The figure shows three views and two pictorial views of one solid part (mm, origin at its lowest corner). Answer the questions. A direction names the side the tool comes from. Give positions to 0.01 mm unless a question says otherwise; leave off trailing zeros. Loops run counter-clockwise (first coordinate to the right, second up) from the corner with the lowest first, then second, coordinate; pieces in that order, holes last. Notation, with made-up numbers: (73.25, 29) - (103.25, 29) arc R18 cw to (103.25, 51) - close; hole circle Ø10 at (74, 47.25). An arc over 180 degrees is marked (long way). Write each question's results on one line, items separated by ' | '.
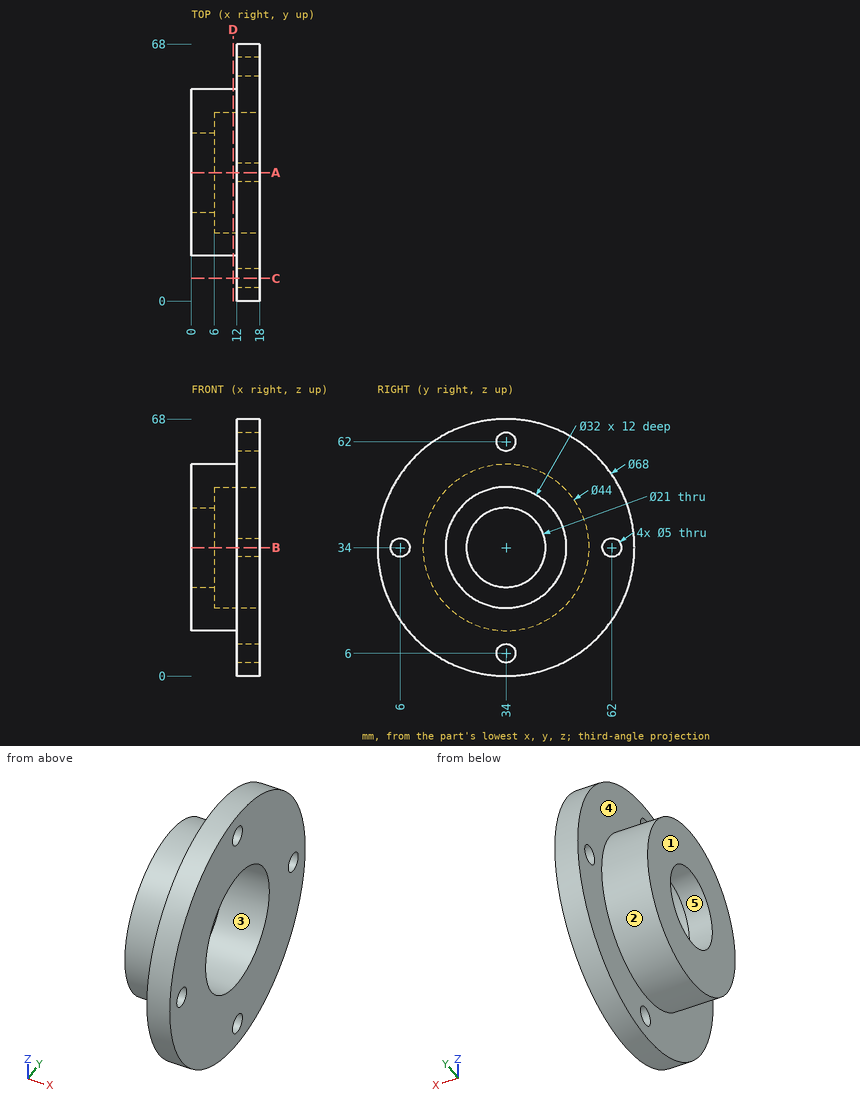
Item 1: Flat-ended cylindrical pins translate along their axes: P1, Ø6, axis at x = 3.5, z = 57, coming from the -Y side; P2, Ø8, axis at x = 6.5, y = 36, coming from the -Z side; P3, Ø1.5, axis at x = 12, y = 44.5, coming from the -Z side; P4, Ø4, axis at y = 6, z = 34, coming from the -X side. Find the tip coordinate at first contact, or state that the pin passes through.
Values found:
P1: stops at y = 24.83 | P2: stops at z = 12 | P3: stops at z = 1.43 | P4: passes through
Item 2: Find the intervals of material crossed by line 1 along Z through (x, y) = (2.25, 34); line 2 along X through (y, z) = (8, 51); line 3 along Y through (x, z) = (12.5, 32.5), in increasing order. Write a range as [from, to].
Values found:
line 1: z = [12, 23.5], [44.5, 56] | line 2: x = [12, 18] | line 3: y = [0.03, 4], [8, 18.07], [49.93, 60], [64, 67.97]
Item 3: A cutting plane is placed at A-A, the plane y = 34. Determine the outline of the cut face in (x, z).
Values found:
outline: (0, 12) - (12, 12) - (12, 8.5) - (18, 8.5) - (18, 18) - (6, 18) - (6, 23.5) - (0, 23.5) - close; (0, 44.5) - (6, 44.5) - (6, 50) - (18, 50) - (18, 59.5) - (12, 59.5) - (12, 56) - (0, 56) - close; (12, 0) - (18, 0) - (18, 3.5) - (12, 3.5) - close; (12, 64.5) - (18, 64.5) - (18, 68) - (12, 68) - close
Item 4: A cutting plane is placed at C-C, the plane y = 6. Determine the outline of the cut face in (x, z).
Values found:
outline: (12, 14.71) - (18, 14.71) - (18, 31.5) - (12, 31.5) - close; (12, 36.5) - (18, 36.5) - (18, 53.29) - (12, 53.29) - close
Item 5: For the marked faces 4 and 5, determine the directions among +Z, -Z, +X, -X, +Y, -Y from which every point of the face is accessible in a straight line to the end or side of a thin tool.
Values found:
face 4: -X | face 5: +X, -X
Item 6: For a pull along Y with two mould halves and no side action, classify the marked faces 1, 2 and 3 as released by +Y, released by -Y, zero draft, split by the parting line, or undercut.
Values found:
face 1: zero draft | face 2: split by the parting line | face 3: undercut
Item 7: A cutting plane is placed at D-D, the plane x = 11. Determine the outline of the cut face in (y, z).
Values found:
outline: circle Ø44 at (34, 34); hole circle Ø32 at (34, 34)
